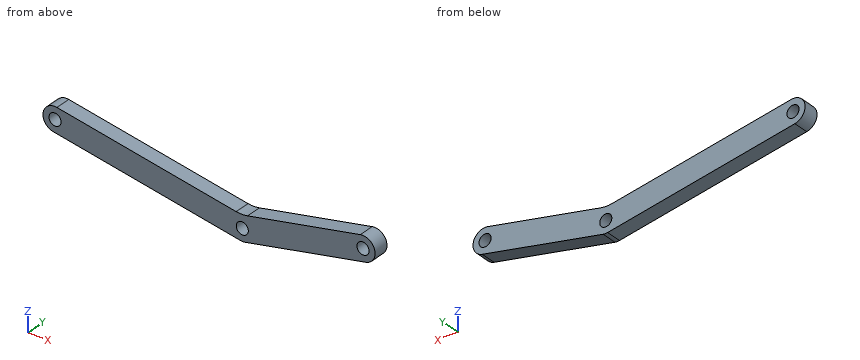
from build123d import *

# Parameters (mm, degrees)
SKETCH_1_R      = 2
EXTRUDE_1_DEPTH = 5
FILLET_2_R      = 10


with BuildPart() as part:
    # 草图1 → 凸台-拉伸1 (new body)
    with BuildSketch(Plane(origin=(0, 0, 0), x_dir=(1, 0, 0), z_dir=(0, 1, 0))):
        with BuildLine():
            Line((10.425672389, 13.301374756), (-51.617327611, 3.955374756))
            ThreePointArc((-51.617327611, 3.955374756), (-54.976874756, -0.595827611), (-50.425672389, -3.955374756))
            Line((-50.425672389, -3.955374756), (10.858587818, 5.276330608))
            Line((10.858587818, 5.276330608), (50.11141182, -3.89509172))
            ThreePointArc((50.11141182, -3.89509172), (54.91659172, -0.91008818), (51.93158818, 3.89509172))
            Line((51.93158818, 3.89509172), (11.93158818, 13.24109172))
            ThreePointArc((11.93158818, 13.24109172), (11.181495117, 13.342798914), (10.425672389, 13.301374756))
        make_face()
        with Locations((-51.0215, 0)):
            Circle(SKETCH_1_R, mode=Mode.SUBTRACT)
        with Locations((11.0215, 9.346)):
            Circle(SKETCH_1_R, mode=Mode.SUBTRACT)
        with Locations((51.0215, 0)):
            Circle(SKETCH_1_R, mode=Mode.SUBTRACT)
    extrude(amount=EXTRUDE_1_DEPTH)

    # 圆角2
    fillet_2_edges = [part.edges().sort_by_distance(p)[0] for p in [
        (10.858587818, 2.5, -5.276330608),
    ]]
    fillet(fillet_2_edges, radius=FILLET_2_R)


solid = part.part
The listing builds one solid part. Answer for the finished solid, in the listing's coordinates (mm). Coordinates: 2 decimals unless noted, no trailing zeros. Order: outer loops, then holes, each group sorted by start corner. A loop starts at its lowest first (then second) coordinate and runs counter-clockwise, first axis right, second up.
Q1. Given P1, Ø2, axis at x = 28, y = 3.5, coming from the -Z side; P2, Ø2.5, axis at x = 11.02, z = -9.35, coming from the +Y side; P3, Ø3, axis at y = 2.5, z = -2.5, coming from the +X side, each flat-ended and moving along its own axis, determine where each tip first touches the part or whether it passes through.
Q2. Consider line 1 (Z direction, x = 49.5, y = 0.8); line 2 (Z direction, x = 12, y = 2.1); line 3 (Z direction, x = 33.5, y = 3.9). Determine where each line is inside the solid, lowest interval first.
Q3. A cutting plane is placed at B-B, the plane y = 2.4. Write down the section's boundary in (x, z).
Q4. A cutting plane is placed at A-A, the plane z = 0. Write down the section's boundary in (x, y), and give its area (3 significant figures).
Q5. A cutting plane is placed at C-C, the plane x = -32.5. Write down the section's boundary in (y, z).
Q6. A cutting plane is placed at D-D, the plane x = 20.5. Write down the section's boundary in (y, z).
Answers follow:
1. P1: stops at z = -9.72
1. P2: passes through
1. P3: stops at x = 54.89
2. line 1: z = -4.46 to -1.3, 1.3 to 3.75
2. line 2: z = -13.23 to -11.09, -7.6 to -4.98
2. line 3: z = -8.2 to 0.01
3. outline: (-51.62, -3.96) - (10.43, -13.3) arc R4 ccw to (11.93, -13.24) - (51.93, -3.9) arc R4 ccw to (50.11, 3.9) - (12.73, -4.84) arc R10 cw to (8.96, -4.99) - (-50.43, 3.96) arc R4 ccw to start; hole circle Ø4 at (-51.02, 0); hole circle Ø4 at (11.02, -9.35); hole circle Ø4 at (51.02, 0)
4. outline: (-55.02, 0) - (-53.02, 0) - (-53.02, 5) - (-55.02, 5) - close; (-49.02, 0) - (-24.17, 0) - (-24.17, 5) - (-49.02, 5) - close; (33.44, 0) - (49.02, 0) - (49.02, 5) - (33.44, 5) - close; (53.02, 0) - (55.02, 0) - (55.02, 5) - (53.02, 5) - close
4. area: 222 mm2
5. outline: (0, -6.84) - (5, -6.84) - (5, 1.26) - (0, 1.26) - close
6. outline: (0, -11.24) - (5, -11.24) - (5, -3.02) - (0, -3.02) - close
